For this review, take the finished solid that the model builds, in its own axes (mm). A direction names the side the tool comes from. Give positions to 0.01 mm unless a question says otherwise; leave off trailing zeros. Write each loop counter-clockwise with the first axis right and the second up, starting at its lowest first coordinate (ties: lowest second). Pieces come first, ordered by that corner, then holes.
Q1. Machinability: for faces 1 (the flat face through (-2, 14, 2)), 2 (the flat face through (0, 54, 0)), which of the approach directions +Z, -Z, +X, -X, +Y, -Y give a long, thin tool a straight path to every point of the face, cutting with its end or side? Answer none if there is none.
Q2. We need section A-A (x = 0). Write out the cut boundary in (y, z).
Q3. For line 1 (Y direction, x = 3, z = 2); line 2 (X direction, y = 11.5, z = -2); line 3 (X direction, y = 43.5, z = 0.5), list the stretches that pass through material, from the lowest coordinate up.
Q4. We need section C-C (z = 0.75). Write out the cut boundary in (x, y).
Q5. Insertion check: P1, Ø1.5, axis at x = 1, y = 37.5, coming from the -Z side; P2, Ø1.4, axis at x = 0, z = 0.5, coming from the -Y side; P3, Ø1.5, axis at x = 3, z = 1.5, coming from the -Y side; P4, Ø2, axis at y = 33.5, z = 1, coming from the -X side. Each pin has a flat end and moves straight along its axis. Give the tip position at first contact, or say it passes through.
Q6. We need section D-D (y = 40). Write out the cut boundary in (x, z).
Q7. We need section B-B (y = 7). Write out the cut boundary in (x, z), then the cut area to 3 significant figures.
Q8. Mouldability with a two-part tool opening along Z and no side actions: class faces 3 (the flat face through (-0.944, 4.437, 0.33)), 4 (the flat face through (-1, 0, 1)), 5 (the flat face through (0, 9, 0)), 6 (the cylindrical face through (2.024, 33.72, 1.29)) as released by +Z, released by -Z, zero draft, split by the parting line, or undercut.
```python
from build123d import *

# Parameters (mm, degrees)
SKETCH2_R           = 4.5
BOSS_EXTRUDE1_DEPTH = 14
CUT_EXTRUDE1_DEPTH  = 9
SKETCH3_R           = 2.4
BOSS_EXTRUDE2_DEPTH = 40


with BuildPart() as part:
    # Sketch2 → Boss-Extrude1 (new body)
    with BuildSketch(Plane(origin=(0, 0, 0), x_dir=(1, 0, 0), z_dir=(0, 1, 0))):
        with Locations(Location((0, 0, 0), (0, 0, 270))):
            Circle(SKETCH2_R)
    extrude(amount=BOSS_EXTRUDE1_DEPTH)

    # Sketch4 → Cut-Extrude1 (cut)
    with BuildSketch(Plane.XZ):
        with BuildLine():
            ThreePointArc((1.5, 0), (0.823094575, 1.253999729), (-0.596687094, 1.376213832))
            Line((-0.596687094, 1.376213832), (-1.301393736, -0.74590505))
            ThreePointArc((-1.301393736, -0.74590505), (0.385946496, -1.449498293), (1.5, 0))
        make_face()
    extrude(amount=-CUT_EXTRUDE1_DEPTH, mode=Mode.SUBTRACT)

    # Sketch3 → Boss-Extrude2 (add)
    with BuildSketch(Plane(origin=(0, 14, 0), x_dir=(1, 0, 0), z_dir=(0, 1, 0))):
        with Locations(Location((0, 0, 0), (0, 0, 270))):
            Circle(SKETCH3_R)
    extrude(amount=BOSS_EXTRUDE2_DEPTH)


solid = part.part
```
Computed:
1. face 1: +Y
1. face 2: +Z, -Z, +X, -X, +Y
2. outline: (0, -4.5) - (14, -4.5) - (14, -2.4) - (54, -2.4) - (54, 2.4) - (14, 2.4) - (14, 4.5) - (0, 4.5) - (0, 1.5) - (9, 1.5) - (9, -1.5) - (0, -1.5) - close
3. line 1: y = 0 to 14
3. line 2: x = -4.03 to 4.03
3. line 3: x = -2.35 to 2.35
4. outline: (-4.44, 0) - (-0.8, 0) - (-0.8, 9) - (1.3, 9) - (1.3, 0) - (4.44, 0) - (4.44, 14) - (2.28, 14) - (2.28, 54) - (-2.28, 54) - (-2.28, 14) - (-4.44, 14) - close
5. P1: stops at z = -2.39
5. P2: stops at y = 9
5. P3: stops at y = 0
5. P4: stops at x = -2.4
6. outline: circle Ø4.8 at (0, 0)
7. outline: circle Ø9 at (0, 0); hole (-1.3, -0.75) arc R1.5 ccw (long way) to (-0.6, 1.38) - close
7. area: 57.3 mm2
8. face 3: undercut
8. face 4: zero draft
8. face 5: undercut
8. face 6: split by the parting line
